```python
from build123d import *

# Parameters (mm, degrees)
F0_W           = 30
F0_H           = 30
F1_DEPTH       = 15
F2_R           = 2
F9_D           = 3
F9_DEPTH       = 1
F9_TIP         = 0.9012909285
F9_ON_F8_D     = 3
F9_ON_F8_DEPTH = 1
F9_ON_F8_TIP   = 0.9012909285
F9_ON_F6_D     = 3
F9_ON_F6_DEPTH = 1
F9_ON_F6_TIP   = 0.9012909285
F9_ON_F7_D     = 3
F9_ON_F7_DEPTH = 1
F9_ON_F7_TIP   = 0.9012909285
F9_ON_F4_D     = 3
F9_ON_F4_DEPTH = 1
F9_ON_F4_TIP   = 0.9012909285
F9_ON_F3_D     = 3
F9_ON_F3_DEPTH = 1
F9_ON_F3_TIP   = 0.9012909285


with BuildPart() as f1:
    # F0 (on Front) → F1 (new body, symmetric)
    with BuildSketch(Plane.XZ):
        Rectangle(F0_W, F0_H)
    extrude(amount=F1_DEPTH, both=True)

    # F2
    f2_edges = [f1.edges().sort_by_distance(p)[0] for p in [
        (0, -15, 15),
        (15, -15, 0),
        (15, 0, 15),
        (0, 15, 15),
        (-15, 0, 15),
        (15, 15, 0),
        (15, 0, -15),
        (0, -15, -15),
        (-15, -15, 0),
        (-15, 15, 0),
        (-15, 0, -15),
        (0, 15, -15),
    ]]
    fillet(f2_edges, radius=F2_R)

    # F9
    with Locations(Plane.YZ.offset(15)):
        with Locations((-10, 10), (-10, -10), (10, 10), (10, -10)):
            Hole(F9_D / 2, depth=F9_DEPTH)
            with Locations((0, 0, -(F9_DEPTH + F9_TIP / 2))):  # 118° drill point
                Cone(0, F9_D / 2, F9_TIP, mode=Mode.SUBTRACT)

    # F9 on F8
    with Locations(Plane(origin=(-15, 0, 0), x_dir=(0, -1, 0), z_dir=(-1, 0, 0))):
        with Locations((0, -10), (0, 10), (10, 10), (-10, 10), (10, -10), (-10, -10)):
            Hole(F9_ON_F8_D / 2, depth=F9_ON_F8_DEPTH)
            with Locations((0, 0, -(F9_ON_F8_DEPTH + F9_ON_F8_TIP / 2))):  # 118° drill point
                Cone(0, F9_ON_F8_D / 2, F9_ON_F8_TIP, mode=Mode.SUBTRACT)

    # F9 on F6
    with Locations(Plane(origin=(0, 15, 0), x_dir=(-1, 0, 0), z_dir=(0, 1, 0))):
        with Locations((10, -10), (-10, 10)):
            Hole(F9_ON_F6_D / 2, depth=F9_ON_F6_DEPTH)
            with Locations((0, 0, -(F9_ON_F6_DEPTH + F9_ON_F6_TIP / 2))):  # 118° drill point
                Cone(0, F9_ON_F6_D / 2, F9_ON_F6_TIP, mode=Mode.SUBTRACT)

    # F9 on F7
    with Locations(Plane.XY.offset(15)):
        with Locations((10, 10), (0, 0), (-10, 10), (10, -10), (-10, -10)):
            Hole(F9_ON_F7_D / 2, depth=F9_ON_F7_DEPTH)
            with Locations((0, 0, -(F9_ON_F7_DEPTH + F9_ON_F7_TIP / 2))):  # 118° drill point
                Cone(0, F9_ON_F7_D / 2, F9_ON_F7_TIP, mode=Mode.SUBTRACT)

    # F9 on F4
    with Locations(Plane(origin=(0, 0, -15), x_dir=(1, 0, 0), z_dir=(0, 0, -1))):
        with Locations((-9.9993329495, -9.9993329495), (9.9993329495, 9.9993329495), (0, 0)):
            Hole(F9_ON_F4_D / 2, depth=F9_ON_F4_DEPTH)
            with Locations((0, 0, -(F9_ON_F4_DEPTH + F9_ON_F4_TIP / 2))):  # 118° drill point
                Cone(0, F9_ON_F4_D / 2, F9_ON_F4_TIP, mode=Mode.SUBTRACT)

    # F9 on F3
    with Locations(Plane.XZ.offset(15)):
        with Locations((0, 0)):
            Hole(F9_ON_F3_D / 2, depth=F9_ON_F3_DEPTH)
            with Locations((0, 0, -(F9_ON_F3_DEPTH + F9_ON_F3_TIP / 2))):  # 118° drill point
                Cone(0, F9_ON_F3_D / 2, F9_ON_F3_TIP, mode=Mode.SUBTRACT)


solid = f1.part
```
Work out the finished part from the listing and answer in its coordinate system (mm). A direction names the side the tool comes from. Round coordinates to 2 decimals unless told otherwise and drop trailing zeros. Write each question's results on one line, items separated by ' | '.
Q1. Straight lines are drawn through the part: line 1 along Y through (x, z) = (10, 14.7); line 2 along Y through (x, z) = (14.45, 10); line 3 along X through (y, z) = (14.65, -10). For each, find the intervals that lie inside material, in ascending order. Write a range as [from, to].
Data:
line 1: [-14.05, -11.5], [-8.5, 8.5], [11.5, 14.05] | line 2: [-14.38, -11.5], [-8.5, 8.5], [11.5, 14.38] | line 3: [-14.13, -11.5], [-8.5, 14.13]
Q2. Flat-ended cylindrical pins translate along their axes: P1, Ø1.8, axis at x = -10, z = -10, coming from the +Y side; P2, Ø2.5, axis at x = -10, y = 10, coming from the -Z side; P3, Ø2.5, axis at y = -10, z = -10, coming from the +X side. Find the tip coordinate at first contact, or state that the pin passes through.
Data:
P1: y = 13.64 | P2: z = -13.85 | P3: x = 13.85
Q3. Which of the six approach directions +Z, -Z, +X, -X, +Y, -Y give full straight-line access (tool end or side, diameter ignored) to faces 1 (the cylindrical face through (11.2, 9.1, 14.5)), 2 (the cylindrical face through (14.5, 11.2, -10.9)), 3 (the cylindrical face through (-14.5, -11.2, 9.1)), 4 (the conical face through (-10.033, 9.741, -13.255))?
Data:
face 1: +Z | face 2: +X | face 3: -X | face 4: -Z
Q4. Determine the mould class of faces 5 (the cylindrical face through (14.43, 14.4, 0.18)), 6 (the conical face through (-13.255, 10.207, -10.159)), 7 (the cylindrical face through (8.8, 14.5, 9.1)) for opening direction Y: released by +Y, released by -Y, zero draft, split by the parting line, or undercut.
Data:
face 5: released by +Y | face 6: undercut | face 7: zero draft
